For this review, take the finished solid that the model builds, in its own axes (mm). Face numbers are marked on the shaded views. A direction names the side the tool comes from. Coordinates: 2 decimals unless noted, no trailing zeros. Order: outer loops, then holes, each group sorted by start corner. A loop starts at its lowest first (then second) coordinate and runs counter-clockwise, first axis right, second up. Notation, with made-up numbers: (3, -35) -> (49, -35) arc R31 cw to (49, -5) -> close; hole circle Ø4 at (72, 83.25). An arc over 180 degrees is marked (long way). Return JSON: item names as keys, results as strings. Group by question number.
Item 1: Take a section at C-C (x = 0). Write out the cut boundary in (y, z), then the cut area to 3 significant figures.
Item 2: Take a section at B-B (z = 0). Write out the cut boundary in (x, y), then the cut area to 3 significant figures.
Item 3: Machinability: for the marked faces 4, 5 and 6, which of the approach directions +Z, -Z, +X, -X, +Y, -Y give a long, thin tool a straight path to every point of the face, cutting with its end or side? Answer none if there is none.
Item 4: Take a section at A-A (y = 4.75). Write out the cut boundary in (x, z).
Item 5: Insertion check: pin 1 (1 mm diameter, centred on y = 0.5, z = 6, fed in from -X); pin 2 (3 mm diameter, centred on x = -20, y = 3.5, fed in from +Z). Each pin has a flat end and moves straight along its axis. Give the tip position at first contact, or say it passes through.
Item 6: Draft analysis for pull direction X (two halves, no side actions). For the marked faces 1, 2 and 3, state which applies: +X half, -X half, draft (parallel to the pull), parting line (faces both ways), or undercut.
Item 7: Take a section at D-D (y = 1.75). Write out the cut boundary in (x, z).
Item 8: For line 1 along Z through (x, y) = (0.5, 2); line 2 along X through (y, z) = (3.5, 0); line 3 along X through (y, z) = (5, 11), list the stretches that pass through material, from the lowest coordinate up.
```python
from build123d import *

# Parameters (mm, degrees)
SKETCH1_R           = 12.7
BOSS_EXTRUDE1_DEPTH = 6.35
CUT_EXTRUDE1_DEPTH  = 2.54


with BuildPart() as part:
    # Sketch1 → Boss-Extrude1 (new body)
    with BuildSketch(Plane(origin=(0, 0, 0), x_dir=(1, 0, 0), z_dir=(0, 1, 0))):
        with BuildLine():
            Line((-21.536991144, 1.27), (-21.536991144, -1.27))
            Line((-21.536991144, -1.27), (-15.186991144, -1.27))
            ThreePointArc((-15.186991144, -1.27), (0, -15.24), (15.186991144, -1.27))
            ThreePointArc((15.186991144, -1.27), (16.408069395, -13.415825599), (19.618283607, -25.193203757))
            Line((19.618283607, -25.193203757), (22.005102864, -24.324472593))
            ThreePointArc((22.005102864, -24.324472593), (17.716042054, 0), (22.005102864, 24.324472593))
            Line((22.005102864, 24.324472593), (19.618283607, 25.193203757))
            ThreePointArc((19.618283607, 25.193203757), (16.408069395, 13.415825599), (15.186991144, 1.27))
            ThreePointArc((15.186991144, 1.27), (0, 15.24), (-15.186991144, 1.27))
            Line((-15.186991144, 1.27), (-21.536991144, 1.27))
        make_face()
        with Locations(Location((0, 0, 0), (0, 0, 270))):
            Circle(SKETCH1_R, mode=Mode.SUBTRACT)
    extrude(amount=BOSS_EXTRUDE1_DEPTH)

    # Sketch2 → Cut-Extrude1 (cut)
    with BuildSketch(Plane(origin=(0, 6.35, 0), x_dir=(1, 0, 0), z_dir=(0, 1, 0))):
        with BuildLine():
            Line((20.428988318, 24.895578462), (21.194398153, 24.622097889))
            ThreePointArc((21.194398153, 24.622097889), (16.927750399, 0), (21.194398153, -24.622097889))
            Line((21.194398153, -24.622097889), (20.428988318, -24.895578462))
            ThreePointArc((20.428988318, -24.895578462), (16.114950399, 0), (20.428988318, 24.895578462))
        make_face()
    extrude(amount=-CUT_EXTRUDE1_DEPTH, mode=Mode.SUBTRACT)


solid = part.part
```
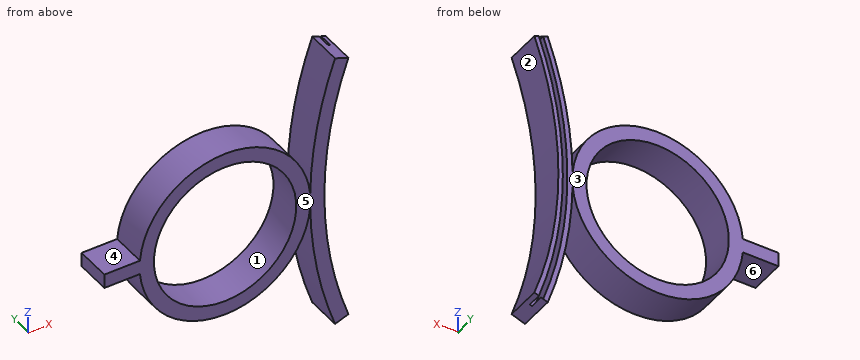
Findings below:
{
 "1": {"outline": "(0, -15.24) -> (6.35, -15.24) -> (6.35, -12.7) -> (0, -12.7) -> close; (0, 12.7) -> (6.35, 12.7) -> (6.35, 15.24) -> (0, 15.24) -> close", "area": "32.3 mm2"},
 "2": {"outline": "(-21.54, 0) -> (-12.7, 0) -> (-12.7, 6.35) -> (-21.54, 6.35) -> close; (12.7, 0) -> (17.72, 0) -> (17.72, 6.35) -> (16.93, 6.35) -> (16.93, 3.81) -> (16.11, 3.81) -> (16.11, 6.35) -> (12.7, 6.35) -> close", "area": "85.9 mm2"},
 "3": {"face 4": "+Z, -X, +Y, -Y", "face 5": "+Z, -Z, +X, -X, -Y", "face 6": "-Z, -X, +Y, -Y"},
 "4": {"outline": "(-21.54, -1.27) -> (-15.19, -1.27) arc R15.24 ccw to (15.19, -1.27) arc R73.66 ccw to (19.62, -25.19) -> (20.81, -24.76) -> (20.43, -24.9) arc R73.99 cw to (20.43, 24.9) -> (20.81, 24.76) -> (19.62, 25.19) arc R73.66 ccw to (15.19, 1.27) arc R15.24 ccw to (-15.19, 1.27) -> (-21.54, 1.27) -> close; (21.19, -24.62) -> (22.01, -24.32) arc R71.12 cw to (22.01, 24.32) -> (21.19, 24.62) arc R73.18 ccw to start; hole circle Ø25.4 at (0, 0)"},
 "5": {"pin 1": "stops at x = -14.21", "pin 2": "stops at z = 1.27"},
 "6": {"face 1": "undercut", "face 2": "+X half", "face 3": "draft"},
 "7": {"outline": "(-21.54, -1.27) -> (-15.19, -1.27) arc R15.24 ccw to (15.19, -1.27) arc R73.66 ccw to (19.62, -25.19) -> (22.01, -24.32) arc R71.12 cw to (22.01, 24.32) -> (19.62, 25.19) arc R73.66 ccw to (15.19, 1.27) arc R15.24 ccw to (-15.19, 1.27) -> (-21.54, 1.27) -> close; hole circle Ø25.4 at (0, 0)"},
 "8": {"line 1": "z = -15.23 to -12.69, 12.69 to 15.23", "line 2": "x = -21.54 to -12.7, 12.7 to 17.72", "line 3": "x = -10.55 to -6.35, 6.35 to 10.55, 16 to 16.94, 17.76 to 18.57"}
}
